Print and shaded views of the part. All mm, measured from the part's lowest x, y and z. A direction names the side the tool comes from. Give positions to 0.01 mm unless a question says otherwise; leave off trailing zeros. Loops run counter-clockwise (first coordinate to the right, second up) from the corner with the lowest first, then second, coordinate; pieces in that order, holes last. Notation, with made-up numbers: (81.25, -28) - (101.25, -28) arc R10 cw to (101.25, -10) - close; hole circle Ø2 at (-23, 70.5). An arc over 180 degrees is marked (long way). Return JSON: item names as keys, results as strings.
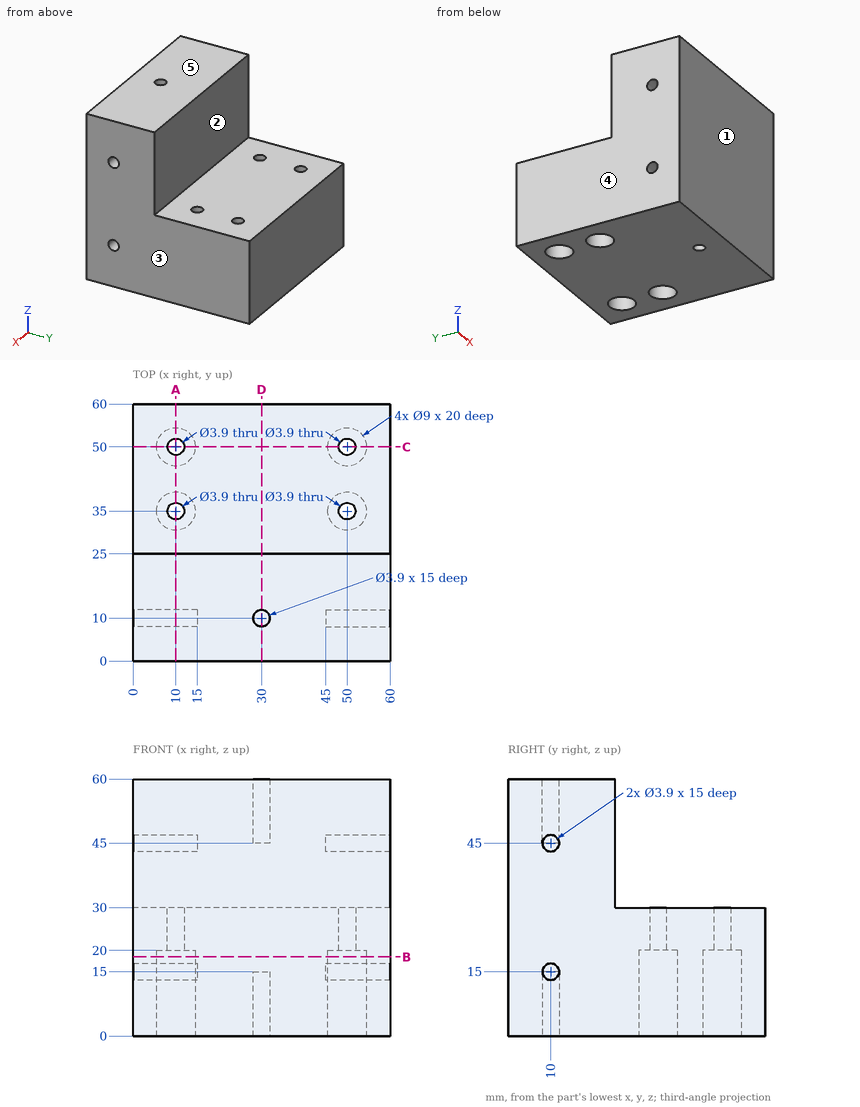
1. Cut at B-B, the plane z = 18.5. Write the cut outline in (x, y).
Values follow:
{"outline": "(0, 0) - (60, 0) - (60, 60) - (0, 60) - close; hole circle Ø9 at (10, 35); hole circle Ø9 at (10, 50); hole circle Ø9 at (50, 35); hole circle Ø9 at (50, 50)"}
2. Which spindle directions (+Z, -Z, +X, -X, +Y, -Y) get a long thin tool onto all of the face, cutting with end or side? Do the marked faces 1 and 2. Say none if no direction does.
Values follow:
{"face 1": "+Z, -Z, +X, -X, -Y", "face 2": "+Z, +X, -X, +Y"}
3. Cut at A-A, the plane x = 10. Write the cut outline in (y, z), plus the area to 3 significant figures.
Values follow:
{"outline": "(0, 0) - (30.5, 0) - (30.5, 20) - (33.05, 20) - (33.05, 30) - (25, 30) - (25, 60) - (0, 60) - close; (36.95, 20) - (39.5, 20) - (39.5, 0) - (45.5, 0) - (45.5, 20) - (48.05, 20) - (48.05, 30) - (36.95, 30) - close; (51.95, 20) - (54.5, 20) - (54.5, 0) - (60, 0) - (60, 30) - (51.95, 30) - close; hole circle Ø3.9 at (10, 15); hole circle Ø3.9 at (10, 45)", "area": "2,090 mm²"}
4. Drill centre lines: probe 1 along Y at (x, z) = (50, 26.75); probe 2 along Y at (x, z) = (10, 6); probe 3 along Z at (x, y) = (49.5, 11). Where is each one in solid material? Low to high.
Values follow:
{"probe 1": "y = 0 to 33.05, 36.95 to 48.05, 51.95 to 60", "probe 2": "y = 0 to 30.5, 39.5 to 45.5, 54.5 to 60", "probe 3": "z = 0 to 13.33, 16.67 to 43.33, 46.67 to 60"}
5. Cut at D-D, the plane x = 30. Write the cut outline in (y, z).
Values follow:
{"outline": "(0, 0) - (8.05, 0) - (8.05, 15) - (11.95, 15) - (11.95, 0) - (60, 0) - (60, 30) - (25, 30) - (25, 60) - (11.95, 60) - (11.95, 45) - (8.05, 45) - (8.05, 60) - (0, 60) - close"}
6. Pull direction X, two halves, no side cores. Call the marked faces 3, 4 and 5: +X half, -X half, draft (parallel to the pull), parting line (faces both ways), or undercut.
Values follow:
{"face 3": "+X half", "face 4": "-X half", "face 5": "draft"}
7. Cut at C-C, the plane y = 50. Write the cut outline in (x, z), plus the area to 3 significant figures.
Values follow:
{"outline": "(0, 0) - (5.5, 0) - (5.5, 20) - (8.05, 20) - (8.05, 30) - (0, 30) - close; (11.95, 20) - (14.5, 20) - (14.5, 0) - (45.5, 0) - (45.5, 20) - (48.05, 20) - (48.05, 30) - (11.95, 30) - close; (51.95, 20) - (54.5, 20) - (54.5, 0) - (60, 0) - (60, 30) - (51.95, 30) - close", "area": "1,360 mm²"}
8. Drop flat-ended pins along their axis: P1, Ø5, axis at x = 50, y = 35, coming from the +Z side; P2, Ø3, axis at x = 30, y = 10, coming from the -Z side; P3, Ø4.5, axis at x = 50.5, y = 33, coming from the -Z side; P4, Ø2, axis at y = 49.5, z = 32.5, coming from the -X side. Give the stop position or say it passes through.
Values follow:
{"P1": "stops at z = 30", "P2": "stops at z = 15", "P3": "stops at z = 20", "P4": "passes through"}
